```python
from build123d import *

# Parameters (mm, degrees)
PAD_DEPTH           = 12
SKETCH001_R         = 2
HOLE_DEPTH          = 5.001
HOLE001_D           = 5
HOLE001_DEPTH       = 25
HOLE001_CSINK_D     = 9
HOLE001_CSINK_ANGLE = 90
FILLET_R            = 2


with BuildPart() as part:
    # Sketch → Pad (new body)
    with BuildSketch(Plane.XY):
        Polygon((0, 15), (0, 0), (15, 0), (15, -5), (-5, -5), (-5, 15), align=None)
    extrude(amount=PAD_DEPTH)

    # Sketch001 (on Face1 of Pad) → Hole (cut, through all)
    with BuildSketch(Plane.YZ):
        with Locations((7, 6)):
            Circle(SKETCH001_R)
    extrude(amount=-HOLE_DEPTH, mode=Mode.SUBTRACT)

    # Hole001
    with Locations(Plane(origin=(0, 0, 0), x_dir=(-1, 0, 0), z_dir=(0, 1, 0))):
        with Locations((-7, 6)):
            CounterSinkHole(HOLE001_D / 2, HOLE001_CSINK_D / 2, depth=HOLE001_DEPTH, counter_sink_angle=HOLE001_CSINK_ANGLE)

    # Fillet
    fillet_edges = [part.edges().sort_by_distance(p)[0] for p in [
        (0, 0, 6),
    ]]
    fillet(fillet_edges, radius=FILLET_R)


solid = part.part
```
Verification items for the finished model (mm, model axes). A direction names the side the tool comes from. Coordinates: 2 decimals unless noted, no trailing zeros. Loops run counter-clockwise (first coordinate to the right, second up) from the corner with the lowest first, then second, coordinate; pieces in that order, holes last. Notation, with made-up numbers: (28.5, 9.5) - (39.5, 9.5) arc R21 cw to (39.5, 26.5) - close; hole circle Ø4 at (83.25, 19.5). An arc over 180 degrees is marked (long way). Answer as a JSON object with one key per item and string values.
(1) Mould release check, pull along X, two halves, no side actions. Record for faces 1 (the cylindrical face through (9.385, -3.521, 6.751)), 2 (the flat face through (-5, 5, 5)), 3 (the flat face through (3, -5, 6)): pulls with the +X half, pulls with the -X half, needs draft (parallel to the pull), parting line crosses it, or undercut.
Response:
{"face 1": "undercut", "face 2": "pulls with the -X half", "face 3": "needs draft"}
(2) Cross-section at C-C, the plane x = 7. Record the boundary of the cut face in (y, z).
Response:
{"outline": "(-5, 0) - (0, 0) - (0, 1.5) - (-2, 3.5) - (-5, 3.5) - close; (-5, 8.5) - (-2, 8.5) - (0, 10.5) - (0, 12) - (-5, 12) - close"}
(3) Cross-section at A-A, the plane y = 7. Record the boundary of the cut face in (x, z), then the cut area to 3 significant figures.
Response:
{"outline": "(-5, 0) - (0, 0) - (0, 4) - (-5, 4) - close; (-5, 8) - (0, 8) - (0, 12) - (-5, 12) - close", "area": "40.0 mm²"}
(4) Scan lines: line 1 along Z through (x, y) = (-1.6, 7); line 2 along X through (y, z) = (-3.3, 6); line 3 along Z through (x, y) = (7, -3.25). Record each from-to range of solid material in increasing order.
Response:
{"line 1": "z = 0 to 4, 8 to 12", "line 2": "x = -5 to 4.5, 9.5 to 15", "line 3": "z = 0 to 3.5, 8.5 to 12"}
(5) Access from +Z, -Z, +X, -X, +Y, -Y to the whole of each face (thin tool, end or side, straight path). Record for faces 4 (the flat face through (11, 0, 3)), 5 (the flat face through (15, -2, 6)).
Response:
{"face 4": "+Z, -Z, +X, +Y", "face 5": "+Z, -Z, +X, +Y, -Y"}
(6) Cross-section at D-D, the plane y = -3.25. Record the boundary of the cut face in (x, z), then the cut area to 3 significant figures.
Response:
{"outline": "(-5, 0) - (15, 0) - (15, 12) - (-5, 12) - close; hole circle Ø5 at (7, 6)", "area": "220 mm²"}
(7) Go/stop test with flat-tipped pins: pin 1 Ø1.5 at (y, z) = (1.5, 8.5) entering from +X; pin 2 Ø3.5 at (y, z) = (8.5, 6.5) entering from +X. Record where each tip stops, or that it passes through.
Response:
{"pin 1": "stops at x = 0.44", "pin 2": "stops at x = 0"}
(8) Cross-section at B-B, the plane z = 6. Record the boundary of the cut face in (x, y).
Response:
{"outline": "(-5, -5) - (4.5, -5) - (4.5, -2) - (2.5, 0) - (2, 0) arc R2 cw to (0, 2) - (0, 5) - (-5, 5) - close; (-5, 9) - (0, 9) - (0, 15) - (-5, 15) - close; (9.5, -5) - (15, -5) - (15, 0) - (11.5, 0) - (9.5, -2) - close"}
